The listing builds one solid part. Answer for the finished solid, in the listing's coordinates (mm). Face numbers are marked on the shaded views. A direction names the side the tool comes from. Coordinates: 2 decimals unless noted, no trailing zeros. Order: outer loops, then holes, each group sorted by start corner. A loop starts at its lowest first (then second) coordinate and runs counter-clockwise, first axis right, second up. Notation, with made-up numbers: (12.5, 49) -> (22.5, 49) arc R15 ccw to (22.5, 59) -> close; hole circle Ø6 at (77.25, -7.75). An arc over 180 degrees is marked (long way). Answer in a Markdown table with one row per item. Add a question column.
```python
from build123d import *

# Parameters (mm, degrees)
BOSS_EXTRUDE4_DEPTH = 6


with BuildPart() as part:
    # Sketch4 → Boss-Extrude4 (new body)
    with BuildSketch(Plane.XY):
        with BuildLine():
            ThreePointArc((0, 21.573833609), (2.244076515, 22.584556995), (3.267964856, 24.822657492))
            ThreePointArc((3.267964856, 24.822657492), (4.865501824, 27.205902748), (7.556485251, 28.201186884))
            ThreePointArc((7.556485251, 28.201186884), (9.568303086, 26.065235227), (9.581188162, 23.131034405))
            ThreePointArc((9.581188162, 23.131034405), (9.348851227, 20.680838348), (10.786916804, 18.683487962))
            ThreePointArc((10.786916804, 18.683487962), (13.235705768, 18.436761833), (15.24146933, 19.86306955))
            ThreePointArc((15.24146933, 19.86306955), (17.816599556, 21.128252), (20.644701633, 20.644701633))
            ThreePointArc((20.644701633, 20.644701633), (21.319011157, 17.789004319), (19.86306955, 15.24146933))
            ThreePointArc((19.86306955, 15.24146933), (18.436761833, 13.235705768), (18.683487962, 10.786916804))
            ThreePointArc((18.683487962, 10.786916804), (20.680838348, 9.348851227), (23.131034405, 9.581188162))
            ThreePointArc((23.131034405, 9.581188162), (25.993753825, 9.389303192), (28.201186884, 7.556485251))
            ThreePointArc((28.201186884, 7.556485251), (27.357307405, 4.74622407), (24.822657492, 3.267964856))
            ThreePointArc((24.822657492, 3.267964856), (22.584556995, 2.244076515), (21.573833609, 0))
            ThreePointArc((21.573833609, 0), (22.584556995, -2.244076515), (24.822657492, -3.267964856))
            ThreePointArc((24.822657492, -3.267964856), (27.205902748, -4.865501824), (28.201186884, -7.556485251))
            ThreePointArc((28.201186884, -7.556485251), (26.065235227, -9.568303086), (23.131034405, -9.581188162))
            ThreePointArc((23.131034405, -9.581188162), (20.680838348, -9.348851227), (18.683487962, -10.786916804))
            ThreePointArc((18.683487962, -10.786916804), (18.436761833, -13.235705768), (19.86306955, -15.24146933))
            ThreePointArc((19.86306955, -15.24146933), (21.128252, -17.816599556), (20.644701633, -20.644701633))
            ThreePointArc((20.644701633, -20.644701633), (17.789004319, -21.319011157), (15.24146933, -19.86306955))
            ThreePointArc((15.24146933, -19.86306955), (13.235705768, -18.436761833), (10.786916804, -18.683487962))
            ThreePointArc((10.786916804, -18.683487962), (9.348851227, -20.680838348), (9.581188162, -23.131034405))
            ThreePointArc((9.581188162, -23.131034405), (9.389303192, -25.993753825), (7.556485251, -28.201186884))
            ThreePointArc((7.556485251, -28.201186884), (4.74622407, -27.357307405), (3.267964856, -24.822657492))
            ThreePointArc((3.267964856, -24.822657492), (2.244076515, -22.584556995), (0, -21.573833609))
            ThreePointArc((0, -21.573833609), (-2.244076515, -22.584556995), (-3.267964856, -24.822657492))
            ThreePointArc((-3.267964856, -24.822657492), (-4.865501824, -27.205902748), (-7.556485251, -28.201186884))
            ThreePointArc((-7.556485251, -28.201186884), (-9.568303086, -26.065235227), (-9.581188162, -23.131034405))
            ThreePointArc((-9.581188162, -23.131034405), (-9.348851227, -20.680838348), (-10.786916804, -18.683487962))
            ThreePointArc((-10.786916804, -18.683487962), (-13.235705768, -18.436761833), (-15.24146933, -19.86306955))
            ThreePointArc((-15.24146933, -19.86306955), (-17.816599556, -21.128252), (-20.644701633, -20.644701633))
            ThreePointArc((-20.644701633, -20.644701633), (-21.319011157, -17.789004319), (-19.86306955, -15.24146933))
            ThreePointArc((-19.86306955, -15.24146933), (-18.436761833, -13.235705768), (-18.683487962, -10.786916804))
            ThreePointArc((-18.683487962, -10.786916804), (-20.680838348, -9.348851227), (-23.131034405, -9.581188162))
            ThreePointArc((-23.131034405, -9.581188162), (-25.993753825, -9.389303192), (-28.201186884, -7.556485251))
            ThreePointArc((-28.201186884, -7.556485251), (-27.357307405, -4.74622407), (-24.822657492, -3.267964856))
            ThreePointArc((-24.822657492, -3.267964856), (-22.584556995, -2.244076515), (-21.573833609, 0))
            ThreePointArc((-21.573833609, 0), (-22.584556995, 2.244076515), (-24.822657492, 3.267964856))
            ThreePointArc((-24.822657492, 3.267964856), (-27.205902748, 4.865501824), (-28.201186884, 7.556485251))
            ThreePointArc((-28.201186884, 7.556485251), (-26.065235227, 9.568303086), (-23.131034405, 9.581188162))
            ThreePointArc((-23.131034405, 9.581188162), (-20.680838348, 9.348851227), (-18.683487962, 10.786916804))
            ThreePointArc((-18.683487962, 10.786916804), (-18.436761833, 13.235705768), (-19.86306955, 15.24146933))
            ThreePointArc((-19.86306955, 15.24146933), (-21.128252, 17.816599556), (-20.644701633, 20.644701633))
            ThreePointArc((-20.644701633, 20.644701633), (-17.789004319, 21.319011157), (-15.24146933, 19.86306955))
            ThreePointArc((-15.24146933, 19.86306955), (-13.235705768, 18.436761833), (-10.786916804, 18.683487962))
            ThreePointArc((-10.786916804, 18.683487962), (-9.348851227, 20.680838348), (-9.581188162, 23.131034405))
            ThreePointArc((-9.581188162, 23.131034405), (-9.389303192, 25.993753825), (-7.556485251, 28.201186884))
            ThreePointArc((-7.556485251, 28.201186884), (-4.74622407, 27.357307405), (-3.267964856, 24.822657492))
            ThreePointArc((-3.267964856, 24.822657492), (-2.244076515, 22.584556995), (0, 21.573833609))
        make_face()
    extrude(amount=BOSS_EXTRUDE4_DEPTH)


solid = part.part
```
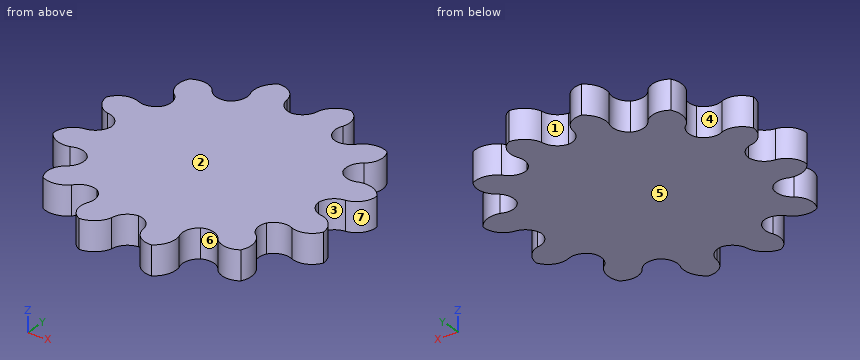
Q1. Determine the mould class of the marked faces 5, 6 and 7 for opening direction X: +X half, -X half, draft (parallel to the pull), parting line (faces both ways), or undercut.
Q2. Given pin 1 (1 mm diameter, centred on x = 0, y = -5.5, fed in from -Z); pin 2 (1.5 mm diameter, centred on y = -18, z = 4.5, fed in from -X); pin 3 (3 mm diameter, centred on y = 11, z = 5, fed in from -X); pin 4 (1.5 mm diameter, centred on x = -6.5, z = 3.5, fed in from -Y), each flat-ended and moving along its own axis, determine where each tip first touches the part or whether it passes through.
Q3. A cutting plane is placed at A-A (y = -4.5). Determine the outline of the cut face in (x, z), then the cut area to 3 significant figures.
Q4. For the marked faces 1, 2, 3 and 4, determine the directions among +Z, -Z, +X, -X, +Y, -Y from which every point of the face is accessible in a straight line to the end or side of a thin tool.
Q5. Straight lines are drawn through the part: line 1 (X direction, y = -20, z = 3.7); line 2 (X direction, y = 12, z = 5.45); line 3 (Y direction, x = 23, z = 2.45). For each, find the intervals that lie inside material, in ascending order.
Returned:
| question | item | result |
|---|---|---|
| 1 | face 5 | draft |
| 1 | face 6 | undercut |
| 1 | face 7 | +X half |
| 2 | pin 1 | stops at z = 0 |
| 2 | pin 2 | stops at x = -21.36 |
| 2 | pin 3 | stops at x = -26.23 |
| 2 | pin 4 | stops at y = -28.18 |
| 3 | outline | (-27.15, 0) -> (26.89, 0) -> (26.89, 6) -> (-27.15, 6) -> close |
| 3 | area | 324 mm² |
| 4 | face 1 | +Z, -Z, +Y |
| 4 | face 2 | +Z, +X, -X, +Y, -Y |
| 4 | face 3 | +Z, -Z, +X |
| 4 | face 4 | +Z, -Z |
| 5 | line 1 | x = -21.01 to -15.39, -9.61 to 9.61, 15.36 to 20.92 |
| 5 | line 2 | x = -18.34 to 18.34 |
| 5 | line 3 | y = -9.52 to -2.6, 2.6 to 9.52 |
